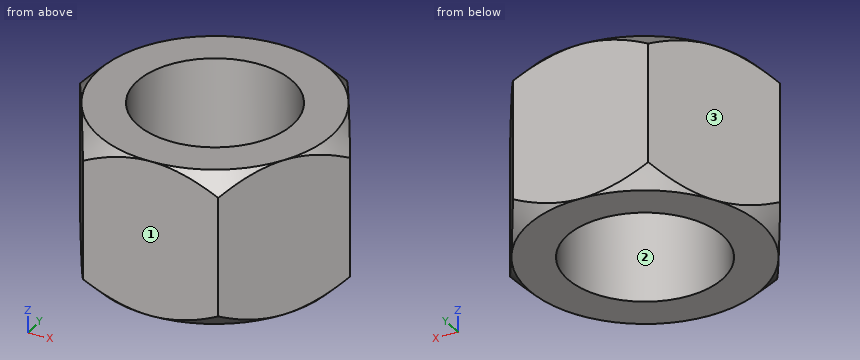
Autodesk Inventor part; units mm, degrees
ref_plane "YZ Plane" through (0, 0, 0) normal (1, 0, 0) x (0, 1, 0)
ref_plane "XZ Plane" through (0, 0, 0) normal (0, 1, 0) x (-1, 0, 0)
ref_plane "XY Plane" through (0, 0, 0) normal (0, 0, 1) x (1, 0, 0)
sketch "Sketch1" plane through (0, 0, 0) normal (0, 0, 1) x (1, 0, 0)
  line L0 (10.3923, 0) -> (5.1962, -9)
  line L1 (5.1962, -9) -> (-5.1962, -9)
  line L2 (-5.1962, -9) -> (-10.3923, 0)
  line L3 (-10.3923, 0) -> (-5.1962, 9)
  line L4 (-5.1962, 9) -> (5.1962, 9)
  line L5 (5.1962, 9) -> (10.3923, 0)
  circle A0 centre (0, 0) radius 6
  dimension "d2" = 18
  dimension "d3" = 12
extrude "Extrusion2" add sketch "Sketch1" along normal blind 12
sketch "Sketch2" plane through (0, 0, 12) normal (0, 0, 1) x (1, 0, 0)
  circle A0 centre (0, 0) radius 6 construction
  circle A1 centre (0, 0) radius 9
  line L0 (-10.3923, 0) -> (-5.1962, -9) construction
extrude "Extrusion3" cut sketch "Sketch2" against normal up to surface (12 mm away) draft 45 keep common part
sketch "Sketch3" plane through (0, 0, 0) normal (0, 0, -1) x (-1, 0, 0)
  circle A0 centre (0, 0) radius 6 construction
  circle A1 centre (0, 0) radius 9
  line L0 (-5.1962, -9) -> (-10.3923, 0) construction
extrude "Extrusion4" cut sketch "Sketch3" against normal up to surface (12 mm away) draft 45 keep common part
thread "Thread1"
equation "\"d3\" = Screw_DIA"
equation "\"d19\" = 55deg"
equation "\"Sketch4_Pitch\" = 1.25"
properties part number "ISO 7040 - M12" material "STEEL, AISI 1015"
Geometry check sheet. Reference: the model listing, model coordinates, mm. Face numbers are marked on the shaded views. Coordinates: 2 decimals unless noted, no trailing zeros. Order: outer loops, then holes, each group sorted by start corner. A loop starts at its lowest first (then second) coordinate and runs counter-clockwise, first axis right, second up. Notation, with made-up numbers: (-10, 44) - (39, 44) arc R16 cw to (39, 75) - close; hole circle Ø3 at (84, 42). An arc over 180 degrees is marked (long way). Answer in a Markdown table with one row per item. Add a question column.
1) Cross-section at A-A, the plane z = 6.25. Record the cut outline in (x, y).
2) Release check for a two-part mould opening along Y. For the marked faces 1, 2 and 3 record: +Y half, -Y half, draft (parallel to the pull), parting line (faces both ways), or undercut.
3) Material ranges on line 1 along Y through (x, z) = (0, 5.25); line 2 along Y through (x, z) = (-4.5, 8.25); line 3 along X through (y, z) = (0.75, 2.75), recorded low to high. Write a range as [from, to].
4) Gauge pin test, flat ends, axial feed: P1, Ø1.5, axis at x = 6, z = 2.5, coming from the +Y side; P2, Ø5, axis at y = -4.5, z = 4, coming from the -X side; P3, Ø4, axis at y = 1, z = 8, coming from the +X side. Record the tip position at first contact, or that the pin passes through.
Check result:
| question | item | result |
|---|---|---|
| 1 | outline | (-10.39, 0) - (-5.2, -9) - (5.2, -9) - (10.39, 0) - (5.2, 9) - (-5.2, 9) - close; hole circle Ø12 at (0, 0) |
| 2 | face 1 | -Y half |
| 2 | face 2 | undercut |
| 2 | face 3 | +Y half |
| 3 | line 1 | y = [-9, -6], [6, 9] |
| 3 | line 2 | y = [-9, -3.97], [3.97, 9] |
| 3 | line 3 | x = [-9.96, -5.95], [5.95, 9.96] |
| 4 | P1 | stops at y = 8.91 |
| 4 | P2 | stops at x = -9.24 |
| 4 | P3 | stops at x = 10.39 |
